Check sheet for the modelled part. Datum: model origin and axes. Units: mm. A direction names the side the tool comes from. Coordinates: 2 decimals unless noted, no trailing zeros. Order: outer loops, then holes, each group sorted by start corner. A loop starts at its lowest first (then second) coordinate and runs counter-clockwise, first axis right, second up. Notation, with made-up numbers: (44.5, 62.5) -> (80.5, 62.5) arc R22 ccw to (80.5, 80.5) -> close; hole circle Ø11 at (83, 22.25). An arc over 180 degrees is marked (long way). Put each result on its own line as item: value. Start each with the question number.
```python
from build123d import *

# Parameters (mm, degrees)
SKETCH1_W               = 80
SKETCH1_H               = 50
BOSS_EXTRUDE1_DEPTH     = 5
SKETCH3_R               = 1.65
CUT_EXTRUDE1_DEPTH      = 5
CUT_EXTRUDE2_DEPTH      = 3
SKETCH5_R               = 1.65
CUT_EXTRUDE3_DEPTH      = 10
MIRROR2_COPY_1_SKETCH_R = 1.65
MIRROR2_COPY_1_DEPTH    = 5
MIRROR2_COPY_2_DEPTH    = 3
MIRROR2_COPY_3_SKETCH_R = 1.65
MIRROR2_COPY_3_DEPTH    = 10
CUT_EXTRUDE4_DEPTH      = 51
SKETCH7_R               = 17.5
CUT_EXTRUDE5_DEPTH      = 7
CUT_EXTRUDE6_DEPTH      = 7


with BuildPart() as part:
    # Sketch1 → Boss-Extrude1 (new body, symmetric)
    with BuildSketch(Plane(origin=(0, 0, 0), x_dir=(1, 0, 0), z_dir=(0, 1, 0))):
        Rectangle(SKETCH1_W, SKETCH1_H)
    extrude(amount=BOSS_EXTRUDE1_DEPTH, both=True)

    # Sketch3 → Cut-Extrude1 (cut)
    with BuildSketch(Plane.XY.offset(25)):
        with Locations((-20, 0)):
            Circle(SKETCH3_R)
    cut_extrude1 = extrude(amount=-CUT_EXTRUDE1_DEPTH, mode=Mode.SUBTRACT)

    # Sketch4 → Cut-Extrude2 (cut)
    with BuildSketch(Plane.XY.offset(20)):
        Polygon((-23, 1.732050808), (-23, 5.757498214), (-17, 5.757498214), (-17, 1.732050808), (-17, -1.732050808), (-20, -3.464101615), (-23, -1.732050808), align=None)
    cut_extrude2 = extrude(amount=-CUT_EXTRUDE2_DEPTH, mode=Mode.SUBTRACT)

    # Sketch5 → Cut-Extrude3 (cut)
    with BuildSketch(Plane.XY.offset(17)):
        with Locations((-20, 0)):
            Circle(SKETCH5_R)
    cut_extrude3 = extrude(amount=-CUT_EXTRUDE3_DEPTH, mode=Mode.SUBTRACT)

    # Mirror1: Cut-Extrude1, Cut-Extrude2, Cut-Extrude3 across plane
    add(cut_extrude1.mirror(Plane(origin=(0, 0, 0), x_dir=(0, 0, 1), z_dir=(1, 0, 0))), mode=Mode.SUBTRACT)
    add(cut_extrude2.mirror(Plane(origin=(0, 0, 0), x_dir=(0, 0, 1), z_dir=(1, 0, 0))), mode=Mode.SUBTRACT)
    add(cut_extrude3.mirror(Plane(origin=(0, 0, 0), x_dir=(0, 0, 1), z_dir=(1, 0, 0))), mode=Mode.SUBTRACT)

    # Mirror2: Cut-Extrude1, Cut-Extrude2, Cut-Extrude3 across plane
    add(cut_extrude1.mirror(Plane.XY), mode=Mode.SUBTRACT)
    add(cut_extrude2.mirror(Plane.XY), mode=Mode.SUBTRACT)
    add(cut_extrude3.mirror(Plane.XY), mode=Mode.SUBTRACT)

    # Mirror2 copy 1 sketch → Mirror2 copy 1 (cut)
    with BuildSketch(Plane(origin=(0, 0, -25), x_dir=(-1, 0, 0), z_dir=(0, 0, -1))):
        with Locations((-20, 0)):
            Circle(MIRROR2_COPY_1_SKETCH_R)
    extrude(amount=-MIRROR2_COPY_1_DEPTH, mode=Mode.SUBTRACT)

    # Mirror2 copy 2 sketch → Mirror2 copy 2 (cut)
    with BuildSketch(Plane(origin=(0, 0, -20), x_dir=(-1, 0, 0), z_dir=(0, 0, -1))):
        Polygon((-23, 1.732050808), (-23, 5.757498214), (-17, 5.757498214), (-17, 1.732050808), (-17, -1.732050808), (-20, -3.464101615), (-23, -1.732050808), align=None)
    extrude(amount=-MIRROR2_COPY_2_DEPTH, mode=Mode.SUBTRACT)

    # Mirror2 copy 3 sketch → Mirror2 copy 3 (cut)
    with BuildSketch(Plane(origin=(0, 0, -17), x_dir=(-1, 0, 0), z_dir=(0, 0, -1))):
        with Locations((-20, 0)):
            Circle(MIRROR2_COPY_3_SKETCH_R)
    extrude(amount=-MIRROR2_COPY_3_DEPTH, mode=Mode.SUBTRACT)

    # Sketch6 → Cut-Extrude4 (cut, through all)
    with BuildSketch(Plane.XY.offset(25)):
        Polygon((-40, 5), (-38.09, 5), (-40, -5), align=None)
    cut_extrude4 = extrude(amount=-CUT_EXTRUDE4_DEPTH, mode=Mode.SUBTRACT)

    # Mirror3: Cut-Extrude4 across plane
    add(cut_extrude4.mirror(Plane(origin=(0, 0, 0), x_dir=(0, 0, 1), z_dir=(1, 0, 0))), mode=Mode.SUBTRACT)

    # Sketch7 → Cut-Extrude5 (cut)
    with BuildSketch(Plane(origin=(0, 5, 0), x_dir=(1, 0, 0), z_dir=(0, 1, 0))):
        Circle(SKETCH7_R)
    extrude(amount=-CUT_EXTRUDE5_DEPTH, mode=Mode.SUBTRACT)

    # Sketch8 → Cut-Extrude6 (cut)
    with BuildSketch(Plane(origin=(0, 5, 0), x_dir=(1, 0, 0), z_dir=(0, 1, 0))):
        with BuildLine():
            Line((22.5, -7.5), (-22.5, -7.5))
            ThreePointArc((-22.5, -7.5), (-30, 0), (-22.5, 7.5))
            Line((-22.5, 7.5), (22.5, 7.5))
            ThreePointArc((22.5, 7.5), (30, 0), (22.5, -7.5))
        make_face()
    extrude(amount=-CUT_EXTRUDE6_DEPTH, mode=Mode.SUBTRACT)


solid = part.part
```
1) Sectioned sample at A-A (z = 14). Record the boundary of the cut face in (x, y), plus the area to 3 significant figures.
2) Sectioned sample at C-C (z = 0). Record the boundary of the cut face in (x, y), plus the area to 3 significant figures.
3) Scan lines: line 1 along X through (y, z) = (-1.5, 16); line 2 along X through (y, z) = (1, 23); line 3 along Y through (x, z) = (20, -22). Record each from-to range of solid material in increasing order. Write a range as [from, to].
4) Mould release check, pull along Z, two halves, no side actions. Record for faces 3 (the flat face through (-1, 0, -25)), 4 (the cylindrical face through (-21.31, -1, -22.54)), 5 (the cylindrical face through (30, 2, 0)): +Z half, -Z half, draft (parallel to the pull), parting line (faces both ways), or undercut.
5) Sectioned sample at D-D (x = -7). Record the boundary of the cut face in (y, z).
6) Access from +Z, -Z, +X, -X, +Y, -Y to the whole of each face (thin tool, end or side, straight path). Record for faces 1 (the flat face through (21.5, -2.6, 18.5)), 2 (the cylindrical face through (-21.31, -1, 22.54)).
7) Gauge pin test, flat ends, axial feed: pin 1 (5 mm diameter, centred on y = 1.5, z = 16, fed in from +X); pin 2 (3.5 mm diameter, centred on y = 3, z = -18.5, fed in from -X); pin 3 (1.5 mm diameter, centred on y = 0.5, z = 18.5, fed in from -X). Record the tip position at first contact, or that the pin passes through.
8) Sectioned sample at B-B (y = 3.5). Record the boundary of the cut face in (x, z), plus the area to 3 significant figures.
Entries:
1. outline: (-40, -5) -> (40, -5) -> (38.09, 5) -> (10.5, 5) -> (10.5, -2) -> (-10.5, -2) -> (-10.5, 5) -> (-38.09, 5) -> close; hole circle Ø3.3 at (-20, 0); hole circle Ø3.3 at (20, 0)
1. area: 617 mm2
2. outline: (-40, -5) -> (40, -5) -> (38.09, 5) -> (30, 5) -> (30, -2) -> (-30, -2) -> (-30, 5) -> (-38.09, 5) -> close
2. area: 361 mm2
3. line 1: x = [-39.33, -20.69], [-19.31, -7.09], [7.09, 19.31], [20.69, 39.33]
3. line 2: x = [-38.85, -21.31], [-18.69, 18.69], [21.31, 38.85]
3. line 3: y = [-5, -1.65], [1.65, 5]
4. face 3: -Z half
4. face 4: draft
4. face 5: undercut
5. outline: (-5, -25) -> (5, -25) -> (5, -16.04) -> (-2, -16.04) -> (-2, 16.04) -> (5, 16.04) -> (5, 25) -> (-5, 25) -> close
6. face 1: +Y
6. face 2: +Z, -Z
7. pin 1: stops at x = 39.24
7. pin 2: stops at x = -38.81
7. pin 3: stops at x = -39.09
8. outline: (-38.38, -25) -> (38.38, -25) -> (38.38, 25) -> (-38.38, 25) -> close; hole (-23, -20) -> (-17, -20) -> (-17, -17) -> (-23, -17) -> close; hole (-23, 17) -> (-17, 17) -> (-17, 20) -> (-23, 20) -> close; hole (-22.5, -7.5) -> (-15.81, -7.5) arc R17.5 ccw to (15.81, -7.5) -> (22.5, -7.5) arc R7.5 ccw to (22.5, 7.5) -> (15.81, 7.5) arc R17.5 ccw to (-15.81, 7.5) -> (-22.5, 7.5) arc R7.5 ccw to start; hole (17, -20) -> (23, -20) -> (23, -17) -> (17, -17) -> close; hole (17, 17) -> (23, 17) -> (23, 20) -> (17, 20) -> close
8. area: 2,460 mm2
